Can you work these out from the model? Positions are in its coordinate system, mm. Give positions to 0.01 mm unless a question says otherwise; leave off trailing zeros. Order: outer loops, then holes, each group sorted by start corner. A loop starts at its lowest first (then second) coordinate and runs counter-clockwise, first axis right, second up.
Item 1: If I drill on line 1 along Z through (x, y) = (1, 9); line 2 along Z through (x, y) = (2.5, 7.5); line 3 along X through (y, z) = (13.5, 14.75) (3 decimals), over which ranges is the centre line in solid material (lowest first)?
Item 2: I want a section at A-A, the plane x = 18.5. Write out the boundary of the cut face in (y, z).
Item 3: I want a section at C-C, the plane y = 8. Write out the boundary of the cut face in (x, z).
Item 4: I'm going to push flat-ended pins straight in: pin 1 Ø6 at (y, z) = (13, 10) entering from -X; pin 2 Ø5 at (x, y) = (3.5, 5.5) entering from +Z; pin 3 Ø3 at (y, z) = (4, 9) entering from -X; pin 4 Ø12 at (x, y) = (2.5, 10) entering from -Z. Where does each tip first touch, or does it pass through?
Item 5: I want a section at B-B, the plane z = 5.5. Write out the boundary of the cut face in (x, y), then the cut area to 3 significant figures.
```python
from build123d import *

# Parameters (mm, degrees)
SKETCH1_W           = 20
SKETCH1_H           = 20
BOSS_EXTRUDE1_DEPTH = 20
CUT_EXTRUDE1_DEPTH  = 20
CUT_EXTRUDE2_DEPTH  = 20


with BuildPart() as part:
    # Sketch1 → Boss-Extrude1 (new body)
    with BuildSketch(Plane.XY):
        with Locations((10, 10)):
            Rectangle(SKETCH1_W, SKETCH1_H)
    extrude(amount=BOSS_EXTRUDE1_DEPTH)

    # Sketch2 → Cut-Extrude1 (cut)
    with BuildSketch(Plane(origin=(0, 20, 0), x_dir=(1, 0, 0), z_dir=(0, 1, 0))):
        Polygon((0, 0), (10, -20), (0, -20), align=None)
    extrude(amount=-CUT_EXTRUDE1_DEPTH, mode=Mode.SUBTRACT)

    # Sketch3 → Cut-Extrude2 (cut)
    with BuildSketch(Plane(origin=(0, 20, 0), x_dir=(1, 0, 0), z_dir=(0, 1, 0))):
        Polygon((20, 0), (10, -20), (20, -20), align=None)
    extrude(amount=-CUT_EXTRUDE2_DEPTH, mode=Mode.SUBTRACT)


solid = part.part
```
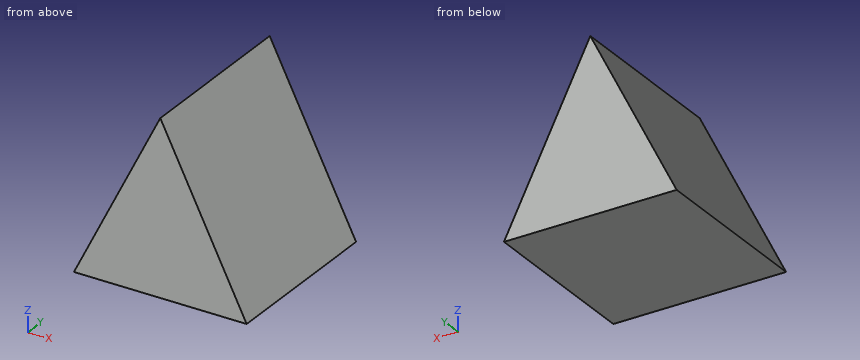
Results list:
1. line 1: z = 0 to 2
1. line 2: z = 0 to 5
1. line 3: x = 7.375 to 12.625
2. outline: (0, 0) - (20, 0) - (20, 3) - (0, 3) - close
3. outline: (0, 0) - (20, 0) - (10, 20) - close
4. pin 1: stops at x = 3.5
4. pin 2: stops at z = 12
4. pin 3: stops at x = 3.75
4. pin 4: stops at z = 0
5. outline: (2.75, 0) - (17.25, 0) - (17.25, 20) - (2.75, 20) - close
5. area: 290 mm2
